Model file for the job. Use its own axes, mm. A direction names the side the tool comes from. Coordinates: 2 decimals unless noted, no trailing zeros. Write each loop counter-clockwise with the first axis right and the second up, starting at its lowest first coordinate (ties: lowest second). Pieces come first, ordered by that corner, then holes. Notation, with made-up numbers: (36.5, -19.75) - (54.5, -19.75) arc R27 cw to (54.5, 0.25) - close; hole circle Ø3 at (-5, -28.75). An arc over 180 degrees is marked (long way). Put each result on its own line as item: value. Start each with the question number.
1. Drop flat-ended pins along their axis: P1, Ø1.8, axis at x = 0, z = 0, coming from the +Y side; P2, Ø5, axis at x = 0, z = 0, coming from the +Y side; P3, Ø4, axis at y = -13, z = -4.5, coming from the +X side; P4, Ø1, axis at x = 5, y = -54, coming from the +Z side. Give the stop position or say it passes through.
2. Saw through at B-B, the plane y = -43.5. Write the cut outline in (x, z).
3. Pull direction Y, two halves, no side cores. Call faces 4 (the face through (0.044, -61.366, -3.745)), 5 (the face through (-3.612, -22.193, 0.802)), 6 (the face through (4, -22.7, -1)), 7 (the face through (0, -5, 0)): released by +Y, released by -Y, zero draft, split by the parting line, or undercut.
4. Saw through at A-A, the plane y = -13.5. Write the cut outline in (x, z).
5. Drill centre lines: L1, parallel to Y at x = 1, z = 7.25; L2, parallel to X at y = -32, z = 0.25; L3, parallel to X at y = -60.75, z = 0. Where is each one in solid material? Low to high. Write a range as from..to.
6. Which spindle directions (+Z, -Z, +X, -X, +Y, -Y) get a long thin tool onto all of the face, cutting with end or side? Do faces 1 (the face through (3, 0, -1)), 2 (the face through (-1, -3, 0)), 3 (the face through (2, -63.7, 2)). Say none if no direction does.
```python
from build123d import *

# Parameters (mm, degrees)
SKETCH_1_R               = 3.9
EXTRUDE_1_DEPTH          = 19
SKETCH_3_R               = 7.7
EXTRUDE_2_DEPTH          = 2.7
SKETCH_4_R               = 3.7
EXTRUDE_3_DEPTH          = 1
SKETCH_5_R               = 4.5
EXTRUDE_4_DEPTH          = 45
CUT_EXTRUDE_1_DEPTH      = 14.75
PATTERN_CIRCULAR_1_COUNT = 4
SKETCH_10_R              = 3.15
CUT_EXTRUDE_2_DEPTH      = 4
CUT_EXTRUDE_START        = -12
SKETCH_11_R              = 2.65
CUT_EXTRUDE_3_DEPTH      = 12
SKETCH_13_R              = 1
SKETCH_12_R              = 2.9
SKETCH_13_2_R            = 1
CUT_EXTRUDE_4_DEPTH      = 3
CHAMFER_1_SIZE           = 0.2


with BuildPart() as part:
    # Эскиз1 → Бобышка-Вытянуть1 (new body)
    with BuildSketch(Plane(origin=(0, 0, 0), x_dir=(1, 0, 0), z_dir=(0, 1, 0))):
        with Locations(Location((0, 0, 0), (0, 0, 270))):
            Circle(SKETCH_1_R)
    extrude(amount=-EXTRUDE_1_DEPTH)

    # Эскиз3 → Бобышка-Вытянуть2 (add)
    with BuildSketch(Plane(origin=(0, -19, 0), x_dir=(1, 0, 0), z_dir=(0, 1, 0))):
        with Locations(Location((0, 0, 0), (0, 0, 270))):
            Circle(SKETCH_3_R)
    extrude(amount=-EXTRUDE_2_DEPTH)

    # Эскиз4 → Бобышка-Вытянуть3 (add)
    with BuildSketch(Plane(origin=(0, -21.7, 0), x_dir=(-1, 0, 0), z_dir=(0, -1, 0))):
        with Locations(Location((0, 0, 0), (0, 0, 90))):
            Circle(SKETCH_4_R)
    extrude(amount=EXTRUDE_3_DEPTH)

    # Эскиз5 → Бобышка-Вытянуть4 (add)
    with BuildSketch(Plane.XZ.offset(22.7)):
        with Locations(Location((0, 0, 0), (0, 0, 90))):
            Circle(SKETCH_5_R)
    extrude(amount=EXTRUDE_4_DEPTH)

    # Эскиз9 → Вырез-Вытянуть1 (cut, symmetric)
    with BuildSketch(Plane.XY):
        Polygon((4.5, -51.7), (3.25, -67.7), (4.5, -67.7), align=None)
    cut_extrude_1 = extrude(amount=CUT_EXTRUDE_1_DEPTH, both=True, mode=Mode.SUBTRACT)

    # Круговой массив1: Вырез-Вытянуть1 ×4 about axis
    pattern_circular_1_axis = Axis((0, 0, 0), (0, 1, 0))
    for i in range(1, PATTERN_CIRCULAR_1_COUNT):
        add(cut_extrude_1.rotate(pattern_circular_1_axis, i * 360 / PATTERN_CIRCULAR_1_COUNT), mode=Mode.SUBTRACT)

    # Эскиз10 → Вырез-Вытянуть2 (cut)
    with BuildSketch(Plane.XZ.offset(67.7)):
        with Locations(Location((0, 0, 0), (0, 0, 270))):
            Circle(SKETCH_10_R)
    extrude(amount=-CUT_EXTRUDE_2_DEPTH, mode=Mode.SUBTRACT)

    # Эскиз11 → Вырез-Вытянуть3 (cut)
    with BuildSketch(Plane.XZ.offset(63.7).offset(CUT_EXTRUDE_START)):
        with Locations(Location((0, 0, 0), (0, 0, 270))):
            Circle(SKETCH_11_R)
    extrude(amount=CUT_EXTRUDE_3_DEPTH, mode=Mode.SUBTRACT)

    # Эскиз13 → Вырез-По сечениям1 section 0
    with BuildSketch(Plane(origin=(0, -2, 0), x_dir=(1, 0, 0), z_dir=(0, 1, 0))):
        Circle(SKETCH_13_R)
    # Эскиз12 → Вырез-По сечениям1 section 1
    with BuildSketch(Plane(origin=(0, 0, 0), x_dir=(1, 0, 0), z_dir=(0, 1, 0))):
        Circle(SKETCH_12_R)
    loft(mode=Mode.SUBTRACT)

    # Эскиз13<2> → Вырез-Вытянуть4 (cut)
    with BuildSketch(Plane(origin=(0, -2, 0), x_dir=(1, 0, 0), z_dir=(0, 1, 0))):
        with Locations(Location((0, 0, 0), (0, 0, 270))):
            Circle(SKETCH_13_2_R)
    extrude(amount=-CUT_EXTRUDE_4_DEPTH, mode=Mode.SUBTRACT)

    # Фаска1
    chamfer_1_edges = [part.edges().sort_by_distance(p)[0] for p in [
        (0, -21.7, -7.7),
        (0, -19, -7.7),
    ]]
    chamfer(chamfer_1_edges, length=CHAMFER_1_SIZE)


solid = part.part
```
Final values:
1. P1: stops at y = -5
1. P2: stops at y = -0.42
1. P3: stops at x = 2.99
1. P4: passes through
2. outline: circle Ø9 at (0, 0)
3. face 4: released by -Y
3. face 5: undercut
3. face 6: undercut
3. face 7: released by +Y
4. outline: circle Ø7.8 at (0, 0)
5. L1: y = -21.7..-19
5. L2: x = -4.49..4.49
5. L3: x = -3.79..-2.65, 2.65..3.79
6. face 1: +Z, -Z, +X, -X, +Y
6. face 2: +Y
6. face 3: -Y
